```python
from build123d import *

# Parameters (mm, degrees)
SKETCH_W     = 400
SKETCH_H     = 30
PAD_DEPTH    = 3
SKETCH001_W  = 270
SKETCH001_H  = 4
POCKET_DEPTH = 3.001


with BuildPart() as part:
    # Sketch → Pad (new body)
    with BuildSketch(Plane.XY):
        with Locations((200, 15)):
            Rectangle(SKETCH_W, SKETCH_H)
    extrude(amount=PAD_DEPTH)

    # Sketch001 → Pocket (cut, through all)
    with BuildSketch(Plane.XY):
        with Locations((145, 15)):
            Rectangle(SKETCH001_W, SKETCH001_H)
        with BuildLine():
            ThreePointArc((295, 21.5), (288.5, 15), (295, 8.5))
            Line((295, 8.5), (385, 8.5))
            ThreePointArc((385, 8.5), (391.5, 15), (385, 21.5))
            Line((295, 21.5), (385, 21.5))
        make_face()
    extrude(amount=POCKET_DEPTH, mode=Mode.SUBTRACT)


solid = part.part
```
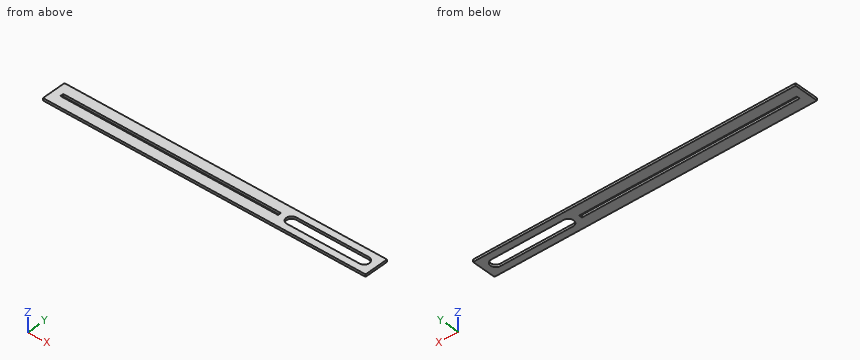
Geometry: final body of the model. Coordinates: model frame, mm. Round coordinates to 2 decimals unless told otherwise and drop trailing zeros. Loops run counter-clockwise (first coordinate to the right, second up) from the corner with the lowest first, then second, coordinate; pieces in that order, holes last. Notation, with made-up numbers: (31.5, -29.5) -> (85.5, -29.5) arc R16 ccw to (85.5, -22.5) -> close; hole circle Ø9 at (16, 62). An arc over 180 degrees is marked (long way). Use one line per item in the form item = value.
Item 1: Cut plane A-A on x = 55. Output: boundary loops of the cut face in (y, z).
Evaluation:
outline = (0, 0) -> (13, 0) -> (13, 3) -> (0, 3) -> close; (17, 0) -> (30, 0) -> (30, 3) -> (17, 3) -> close
Item 2: Material intervals for probe 1 along X at (y, z) = (14, 0.55); probe 2 along X at (y, z) = (15.5, 2.05); probe 3 along Y at (x, z) = (166.5, 2.15), sorted ascending.
Evaluation:
probe_1 = 0 to 10, 280 to 288.58, 391.42 to 400
probe_2 = 0 to 10, 280 to 288.52, 391.48 to 400
probe_3 = 0 to 13, 17 to 30
Item 3: Cut plane B-B on z = 2.35. Output: boundary loops of the cut face in (x, y), then the cut area to 3 significant figures.
Evaluation:
outline = (0, 0) -> (400, 0) -> (400, 30) -> (0, 30) -> close; hole (10, 13) -> (280, 13) -> (280, 17) -> (10, 17) -> close; hole (295, 8.5) -> (385, 8.5) arc R6.5 ccw to (385, 21.5) -> (295, 21.5) arc R6.5 ccw to start
area = 9,620 mm2
Item 4: Cut plane C-C on x = 345. Output: boundary loops of the cut face in (y, z), then the cut area to 3 significant figures.
Evaluation:
outline = (0, 0) -> (8.5, 0) -> (8.5, 3) -> (0, 3) -> close; (21.5, 0) -> (30, 0) -> (30, 3) -> (21.5, 3) -> close
area = 51.0 mm2
